Here's how the part is built. I have some questions about the finished solid (model axes, mm). Face numbers are marked on the shaded views. A direction names the side the tool comes from. Coordinates: 2 decimals unless noted, no trailing zeros. Loops run counter-clockwise (first coordinate to the right, second up) from the corner with the lowest first, then second, coordinate; pieces in that order, holes last. Notation, with made-up numbers: (39.25, -17) - (52.25, -17) arc R26 ccw to (52.25, 9) - close; hole circle Ø8 at (74.25, 3). An arc over 180 degrees is marked (long way). Use a Markdown table: item, result.
```python
from build123d import *

# Parameters (mm, degrees)
F0_R     = 37.5
F1_DEPTH = 70
F2_R     = 10
F3_DEPTH = 35
F5_DEPTH = 35
F7_W     = 50
F7_H     = 10
F6_DEPTH = 40


with BuildPart() as f1:
    # F0 (on Top) → F1 (new body)
    with BuildSketch(Plane.XY):
        Circle(F0_R)
    extrude(amount=F1_DEPTH)

    # F2 (on face) → F3 (cut)
    with BuildSketch(Plane(origin=(0, 0, 0), x_dir=(1, 0, 0), z_dir=(0, 0, -1))):
        Circle(F2_R)
    extrude(amount=-F3_DEPTH, mode=Mode.SUBTRACT)

    # F4 (on face) → F5 (cut)
    with BuildSketch(Plane.XY.offset(70)):
        Polygon((0, 17.5), (-20, -17.141016), (20, -17.141016), align=None)
    extrude(amount=-F5_DEPTH, mode=Mode.SUBTRACT)

    # F7 (on Front) → F6 (cut, symmetric)
    with BuildSketch(Plane.XZ):
        with Locations((0.330579, 14.619615)):
            Rectangle(F7_W, F7_H)
    extrude(amount=F6_DEPTH, both=True, mode=Mode.SUBTRACT)


solid = f1.part
```
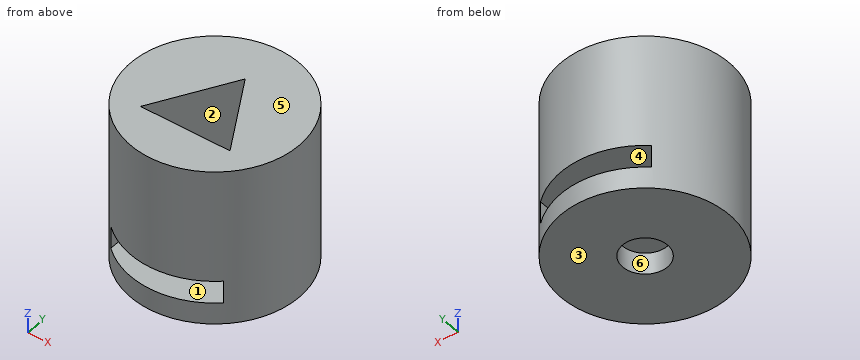
Q1. Which directions (+Z, -Z, +X, -X, +Y, -Y) give clear straight access to the entire face, cutting with the end or side of a thin tool? Please do the marked faces 5 and 6.
Check values:
| item | result |
|---|---|
| face 5 | +Z, +X, -X, +Y, -Y |
| face 6 | -Z |
Q2. I want a section at B-B, the plane y = -1.5. Write out the boundary of the cut face in (x, z), then the cut area to 3 significant figures.
Check values:
| item | result |
|---|---|
| outline | (-37.47, 0) - (-9.89, 0) - (-9.89, 9.62) - (-24.67, 9.62) - (-24.67, 19.62) - (-9.89, 19.62) - (-9.89, 35) - (-10.97, 35) - (-10.97, 70) - (-37.47, 70) - close; (9.89, 0) - (37.47, 0) - (37.47, 70) - (10.97, 70) - (10.97, 35) - (9.89, 35) - (9.89, 19.62) - (25.33, 19.62) - (25.33, 9.62) - (9.89, 9.62) - close |
| area | 3,480 mm^2 |
Q3. Will these pins go through, and if not, where does the flat tip stop? P1, Ø8, axis at x = -3.5, z = 12.5, coming from the +Y side; P2, Ø1.5, axis at y = 6.5, z = 13.5, coming from the +X side; P3, Ø5, axis at x = -9.5, y = -8, coming from the +Z side; P4, Ø16, axis at x = 0, y = 0, coming from the +Z side.
Check values:
| item | result |
|---|---|
| P1 | y = 37.49 |
| P2 | x = 37.06 |
| P3 | z = 35 |
| P4 | through |
Q4. I want a section at A-A, the plane x = 2.5. Write out the boundary of the cut face in (y, z).
Check values:
| item | result |
|---|---|
| outline | (-37.42, 0) - (-9.68, 0) - (-9.68, 9.62) - (-37.42, 9.62) - close; (-37.42, 19.62) - (-9.68, 19.62) - (-9.68, 35) - (-17.14, 35) - (-17.14, 70) - (-37.42, 70) - close; (9.68, 0) - (37.42, 0) - (37.42, 9.62) - (9.68, 9.62) - close; (9.68, 19.62) - (37.42, 19.62) - (37.42, 70) - (13.17, 70) - (13.17, 35) - (9.68, 35) - close |
Q5. I want a section at C-C, the plane x = -18. Write out the boundary of the cut face in (y, z).
Check values:
| item | result |
|---|---|
| outline | (-32.9, 0) - (32.9, 0) - (32.9, 9.62) - (-32.9, 9.62) - close; (-32.9, 19.62) - (32.9, 19.62) - (32.9, 70) - (-13.68, 70) - (-13.68, 35) - (-17.14, 35) - (-17.14, 70) - (-32.9, 70) - close |
Q6. Please list where these lines run through material, in increasing order: L1, parallel to Z at x = -18.5, y = -14; L2, parallel to Z at x = 3, y = -15; L3, parallel to Y at x = 0, z = 7. Write a range as from..to.
Check values:
| item | result |
|---|---|
| L1 | 0..9.62, 19.62..70 |
| L2 | 0..9.62, 19.62..35 |
| L3 | -37.5..-10, 10..37.5 |
Q7. If we mould it in two halves opening along Z, with no side actions, what happens to the marked faces 1, 2, 3 and 4? For each: pulls with the +Z half, pulls with the -Z half, needs draft (parallel to the pull), parting line crosses it, or undercut.
Check values:
| item | result |
|---|---|
| face 1 | undercut |
| face 2 | needs draft |
| face 3 | pulls with the -Z half |
| face 4 | undercut |
Q8. I want a section at D-D, the plane z = 47.5. Write out the boundary of the cut face in (x, y), then the cut area to 3 significant figures.
Check values:
| item | result |
|---|---|
| outline | circle Ø75 at (0, 0); hole (-20, -17.14) - (20, -17.14) - (0, 17.5) - close |
| area | 3,730 mm^2 |
